Design review of the part built by this model. Coordinates are the model's own, in mm. Face numbers are marked on the shaded views. A direction names the side the tool comes from. Give positions to 0.01 mm unless a question says otherwise; leave off trailing zeros. Write each loop counter-clockwise with the first axis right and the second up, starting at its lowest first coordinate (ties: lowest second). Pieces come first, ordered by that corner, then holes. Notation, with made-up numbers: (58, 44) -> (107, 44) arc R22 ccw to (107, 76) -> close; hole circle Ø3 at (17.5, -29.75). An arc over 180 degrees is marked (long way). Answer as a JSON object with one key per item and string values.
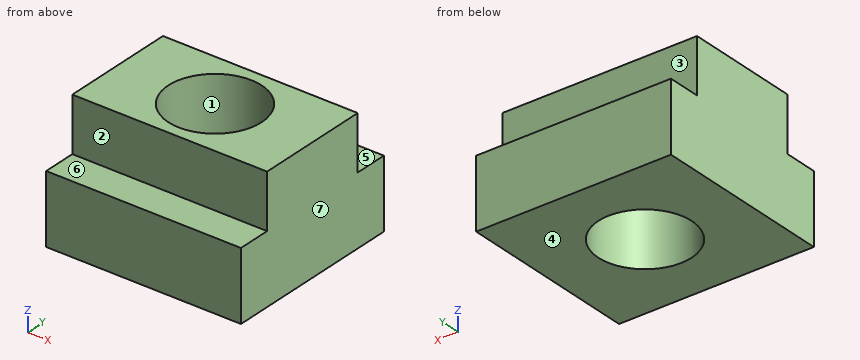
```python
from build123d import *

# Parameters (mm, degrees)
F1_DEPTH = 29.75
F2_R     = 7.125
F3_DEPTH = 18.901


with BuildPart() as f1:
    # F0 (on Right) → F1 (new body)
    with BuildSketch(Plane.YZ):
        Polygon((8.85, 0), (-8.85, 0), (-8.85, -8.3), (-13.95, -8.3), (-13.95, -18.9), (13.95, -18.9), (13.95, -8.3), (8.85, -8.3), align=None)
    extrude(amount=F1_DEPTH)

    # F2 (on face) → F3 (cut, through all)
    with BuildSketch(Plane.XY):
        with Locations((14.875, 0)):
            Circle(F2_R)
    extrude(amount=-F3_DEPTH, mode=Mode.SUBTRACT)


solid = f1.part
```
(1) Clearance check with flat-ended pins moving along their axes: pin 1 (2.5 mm diameter, centred on x = 16, y = -11, fed in from +Z); pin 2 (3 mm diameter, centred on x = 13, z = -2, fed in from +Y); pin 3 (6.5 mm diameter, centred on x = 9.5, z = -5, fed in from -Y). State where each tip first meets the part, or that it passes through.
Here are the results:
{"pin 1": "stops at z = -8.3", "pin 2": "stops at y = 8.85", "pin 3": "stops at y = -8.85"}
(2) We need section C-C, the plane x = 5. State the section outline as (y, z) points, then the cut area to 3 significant figures.
Here are the results:
{"outline": "(-13.95, -18.9) -> (13.95, -18.9) -> (13.95, -8.3) -> (8.85, -8.3) -> (8.85, 0) -> (-8.85, 0) -> (-8.85, -8.3) -> (-13.95, -8.3) -> close", "area": "443 mm²"}
(3) For the marked faces 5, 6 and 7, list the 3-axis set-ups (+Z, -Z, +X, -X, +Y, -Y) from which the entire face can be reached by the end or side of a thin tool; tool diameter is ignored.
Here are the results:
{"face 5": "+Z, +X, -X, +Y", "face 6": "+Z, +X, -X, -Y", "face 7": "+Z, -Z, +X, +Y, -Y"}
(4) We need section D-D, the plane x = 12.75. State the section outline as (y, z) points, then the cut area to 3 significant figures.
Here are the results:
{"outline": "(-13.95, -18.9) -> (-6.8, -18.9) -> (-6.8, 0) -> (-8.85, 0) -> (-8.85, -8.3) -> (-13.95, -8.3) -> close; (6.8, -18.9) -> (13.95, -18.9) -> (13.95, -8.3) -> (8.85, -8.3) -> (8.85, 0) -> (6.8, 0) -> close", "area": "186 mm²"}
(5) For line 1 along X through (y, z) = (4.75, -13.5); line 2 along Y through (x, z) = (18.25, -3.25); line 3 along Z through (x, y) = (15, -11.25), list the stretches that pass through material, from the lowest coordinate up.
Here are the results:
{"line 1": "x = 0 to 9.56, 20.19 to 29.75", "line 2": "y = -8.85 to -6.27, 6.27 to 8.85", "line 3": "z = -18.9 to -8.3"}
(6) The part is to be moulded in two halves that separate along Y. For the marked faces 1, 2, 3 and 4, say which applies: +Y half, -Y half, draft (parallel to the pull), parting line (faces both ways), or undercut.
Here are the results:
{"face 1": "undercut", "face 2": "-Y half", "face 3": "+Y half", "face 4": "draft"}
(7) We need section B-B, the plane z = -3.5. State the section outline as (x, y) points (3 decimals).
Here are the results:
{"outline": "(0, -8.85) -> (29.75, -8.85) -> (29.75, 8.85) -> (0, 8.85) -> close; hole circle Ø14.25 at (14.875, 0)"}
(8) We need section A-A, the plane y = 0. State the section outline as (x, z) points, then the cut area to 3 significant figures.
Here are the results:
{"outline": "(0, -18.9) -> (7.75, -18.9) -> (7.75, 0) -> (0, 0) -> close; (22, -18.9) -> (29.75, -18.9) -> (29.75, 0) -> (22, 0) -> close", "area": "293 mm²"}
